Part model, mm, in its own coordinate system. Coordinates: 2 decimals unless noted, no trailing zeros. Loops run counter-clockwise (first coordinate to the right, second up) from the corner with the lowest first, then second, coordinate; pieces in that order, holes last. Notation, with made-up numbers: (65.5, -21.75) - (73.5, -21.75) arc R24 cw to (73.5, -9.75) - close; hole circle Ø5 at (-10, 52). An arc over 180 degrees is marked (long way). Use a Markdown table: item, result. Add a question column.
1) Probe probe 1 along Y at (x, z) = (-2.5, 3.5); probe 2 along X at (y, z) = (1.4, 0); probe 3 along X at (y, z) = (2.9, 0). List the from-to ranges inside material, lowest first. Write a range as [from, to].
2) Band-saw the part on C-C (y = 2.5). Give the cut face in (x, z).
3) Band-saw the part on D-D (y = 6.5). Give the cut face in (x, z), plus the area to 3 significant figures.
4) Pull direction Z, two halves, no side cores. Call faces 1 (the face through (-4.66, 0.84, -0.61)), 2 (the face through (2.601, 5.477, -0.578)), 3 (the face through (2, 0, -2)), 4 (the face through (-2.52, 2.7, -0.33)): +Z half, -Z half, draft (parallel to the pull), parting line (faces both ways), or undercut.
5) Band-saw the part on B-B (x = 0). Give the cut face in (y, z) (3 decimals), plus the area to 3 significant figures.
6) Drop flat-ended pins along their axis: P1, Ø4, axis at x = -2.5, y = 4, coming from the +Z side; P2, Ø1.5, axis at y = 6.5, z = 1, coming from the +X side; P3, Ø2, axis at y = 6, z = -2, coming from the -X side. Give the stop position or say it passes through.
7) Band-saw the part on A-A (z = 0). Give the cut face in (x, y) (3 decimals).
from build123d import *


with BuildPart() as part:
    # Sketch1 → Revolve1 (revolve)
    with BuildSketch(Plane.XY, mode=Mode.PRIVATE) as revolve1_sk:
        with BuildLine():
            Line((0, 0), (4.699, 0))
            Line((4.699, 0), (4.699, 1.656784628))
            ThreePointArc((4.699, 1.656784628), (3.621369312, 2.103153847), (3.175, 3.180784498))
            ThreePointArc((3.175, 3.180784498), (3.580954352, 4.767014148), (4.699, 5.963215372))
            Line((4.699, 5.963215372), (4.699, 7.62))
            Line((4.699, 7.62), (0, 7.62))
            Line((0, 7.62), (0, 0))
        make_face()
    revolve(revolve1_sk.sketch.rotate(Axis((0, 7.62, 0), (0, -1, 0)), 90), axis=Axis((0, 7.62, 0), (0, -1, 0)))

    # Sketch2 → Cut-Revolve1 (revolve, cut)
    with BuildSketch(Plane.XY, mode=Mode.PRIVATE) as cut_revolve1_sk:
        Polygon((0, 0), (2.54, 0), (2.54, 5.334), (4.527189483, 7.62), (0, 7.62), align=None)
    revolve(cut_revolve1_sk.sketch.rotate(Axis((0, 7.62, 0), (0, -1, 0)), 90), axis=Axis((0, 7.62, 0), (0, -1, 0)), mode=Mode.SUBTRACT)


solid = part.part
Answer block:
| question | item | result |
|---|---|---|
| 1 | probe 1 | [0, 1.71], [5.66, 7.36] |
| 1 | probe 2 | [-4.7, -2.54], [2.54, 4.7] |
| 1 | probe 3 | [-3.2, -2.54], [2.54, 3.2] |
| 2 | outline | circle Ø6.67 at (0, 0); hole circle Ø5.08 at (0, 0) |
| 3 | outline | circle Ø9.4 at (0, 0); hole circle Ø7.11 at (0, 0) |
| 3 | area | 29.7 mm2 |
| 4 | face 1 | parting line |
| 4 | face 2 | undercut |
| 4 | face 3 | draft |
| 4 | face 4 | undercut |
| 5 | outline | (0, -4.699) - (1.657, -4.699) arc R1.524 cw to (3.181, -3.175) arc R3.302 cw to (5.963, -4.699) - (7.62, -4.699) - (7.62, -4.527) - (5.334, -2.54) - (0, -2.54) - close; (0, 2.54) - (5.334, 2.54) - (7.62, 4.527) - (7.62, 4.699) - (5.963, 4.699) arc R3.302 cw to (3.181, 3.175) arc R1.524 cw to (1.657, 4.699) - (0, 4.699) - close |
| 5 | area | 18.7 mm2 |
| 6 | P1 | z = 4.21 |
| 6 | P2 | x = 4.69 |
| 6 | P3 | x = -4.59 |
| 7 | outline | (-4.699, 0) - (-2.54, 0) - (-2.54, 5.334) - (-4.527, 7.62) - (-4.699, 7.62) - (-4.699, 5.963) arc R3.302 cw to (-3.175, 3.181) arc R1.524 cw to (-4.699, 1.657) - close; (2.54, 0) - (4.699, 0) - (4.699, 1.657) arc R1.524 cw to (3.175, 3.181) arc R3.302 cw to (4.699, 5.963) - (4.699, 7.62) - (4.527, 7.62) - (2.54, 5.334) - close |
